Verification items for the finished model (mm, model axes). Give positions to 0.01 mm unless a question says otherwise; leave off trailing zeros. Write each loop counter-clockwise with the first axis right and the second up, starting at its lowest first coordinate (ties: lowest second). Pieces come first, ordered by that corner, then holes. Notation, with made-up numbers: (43.25, -20) - (58.25, -20) arc R20 ccw to (58.25, 12) - close; hole circle Ø7 at (-22.5, -25.5). An arc over 180 degrees is marked (long way). Answer as a JSON object with one key per item and string values. Group by question number.
Item 1: Go/stop test with flat-tipped pins: pin 1 (1.2 mm diameter, centred on x = 2.5, z = -26.5, fed in from -Y); pin 2 (2 mm diameter, centred on x = 1.5, z = -142, fed in from +Y); pin 3 (5 mm diameter, centred on y = 14, z = -33, fed in from -X); pin 4 (2 mm diameter, centred on x = 0.5, z = -36.5, fed in from +Y). Record where each tip stops, or that it passes through.
Item 2: Sectioned sample at B-B, the plane x = 2.8. Record the boundary of the cut face in (y, z), and give its area (3 significant figures).
Item 3: Sectioned sample at D-D, the plane z = 15.5. Record the boundary of the cut face in (x, y).
Item 4: Sectioned sample at A-A, the plane y = 88.9. Record the boundary of the cut face in (x, z), and give its area (3 significant figures).
Item 5: Scan lines: line 1 along Z through (x, y) = (2.35, 88.9); line 2 along Z through (x, y) = (0.6, 25.5); line 3 along Z through (x, y) = (2.65, 115). Record each from-to range of solid material in increasing order. Write a range as [from, to].
Item 6: Draft check along Z on faces 1 (the face through (4.089, 20, -26)), 2 (the face through (2.016, 149.972, 45.235)), 3 (the face through (2.02, 158.74, 43.47)). Enter one of: +Z half, -Z half, draft (parallel to the pull), parting line (faces both ways), or undercut.
Item 7: Sectioned sample at C-C, the plane z = 44.45. Record the boundary of the cut face in (x, y).
```python
from build123d import *

# Parameters (mm, degrees)
F0_R     = 15.621
F0_W     = 5.08
F0_H     = 4.0894
F0_W_2   = 4.826
F1_DEPTH = 4.0894
F2_W     = 5.08
F2_H     = 4.0894
F3_DEPTH = 25.4


with BuildPart() as f1:
    # F0 (on Right) → F1 (new body)
    with BuildSketch(Plane.YZ):
        with BuildLine():
            Line((53.34, -139.7), (114.3, -139.7))
            Line((114.3, -139.7), (114.3, 0))
            Line((114.3, 0), (114.3, 8.769464))
            Line((114.3, 8.769464), (114.3, 80.130536))
            Line((114.3, 80.130536), (114.3, 88.9))
            Line((114.3, 88.9), (-42.671357, 88.9))
            ThreePointArc((-42.671357, 88.9), (-96.063758, -19.892153), (-114.3, -139.7))
            Line((-114.3, -139.7), (-53.34, -139.7))
            Line((-53.34, -139.7), (-48.26, -139.7))
            Line((-48.26, -139.7), (-2.413, -139.7))
            Line((-2.413, -139.7), (2.413, -139.7))
            Line((2.413, -139.7), (48.26, -139.7))
            Line((48.26, -139.7), (53.34, -139.7))
        make_face()
        with Locations((88.9, 44.45)):
            Circle(F0_R, mode=Mode.SUBTRACT)
        with Locations((50.8, -141.7447)):
            Rectangle(F0_W, F0_H)
        with BuildLine():
            Line((114.3, 8.769464), (114.3, 0))
            ThreePointArc((114.3, 0), (158.75, 44.45), (114.3, 88.9))
            Line((114.3, 88.9), (114.3, 80.130536))
            ThreePointArc((114.3, 80.130536), (149.980536, 44.45), (114.3, 8.769464))
        make_face()
        with Locations((0, -141.7447)):
            Rectangle(F0_W_2, F0_H)
        with Locations((-50.8, -141.7447)):
            Rectangle(F0_W, F0_H)
    extrude(amount=F1_DEPTH)

    # F2 (on face) → F3 (cut)
    with BuildSketch(Plane.YZ.offset(4.0894)):
        with Locations((0, -27.4447)):
            Rectangle(F2_W, F2_H)
        with Locations((-25.4, -27.4447)):
            Rectangle(F2_W, F2_H)
    extrude(amount=-F3_DEPTH, mode=Mode.SUBTRACT)


solid = f1.part
```
Geometry check:
{
 "1": {"pin 1": "y = -98.25", "pin 2": "y = 53.34", "pin 3": "x = 0", "pin 4": "y = 114.3"},
 "2": {"outline": "(-114.3, -139.7) - (-53.34, -139.7) - (-53.34, -143.79) - (-48.26, -143.79) - (-48.26, -139.7) - (-2.41, -139.7) - (-2.41, -143.79) - (2.41, -143.79) - (2.41, -139.7) - (48.26, -139.7) - (48.26, -143.79) - (53.34, -143.79) - (53.34, -139.7) - (114.3, -139.7) - (114.3, 0) arc R44.45 ccw to (114.3, 88.9) - (-42.67, 88.9) arc R398.64 ccw to start; hole (-27.94, -29.49) - (-22.86, -29.49) - (-22.86, -25.4) - (-27.94, -25.4) - close; hole (-2.54, -29.49) - (2.54, -29.49) - (2.54, -25.4) - (-2.54, -25.4) - close; hole circle Ø31.24 at (88.9, 44.45); hole (114.3, 8.77) arc R35.68 ccw to (114.3, 80.13) - close", "area": "47,400 mm^2"},
 "3": {"outline": "(0, -83.11) - (4.09, -83.11) - (4.09, 114.3) - (0, 114.3) - close; (0, 135.16) - (4.09, 135.16) - (4.09, 148.03) - (0, 148.03) - close"},
 "4": {"outline": "(0, -139.7) - (4.09, -139.7) - (4.09, 28.83) - (0, 28.83) - close; (0, 60.07) - (4.09, 60.07) - (4.09, 88.9) - (0, 88.9) - close", "area": "807 mm^2"},
 "5": {"line 1": "[-139.7, 28.83], [60.07, 88.9]", "line 2": "[-139.7, 88.9]", "line 3": "[0.01, 8.78], [80.12, 88.89]"},
 "6": {"face 1": "draft", "face 2": "undercut", "face 3": "parting line"},
 "7": {"outline": "(0, -69.54) - (4.09, -69.54) - (4.09, 73.28) - (0, 73.28) - close; (0, 104.52) - (4.09, 104.52) - (4.09, 114.3) - (0, 114.3) - close; (0, 149.98) - (4.09, 149.98) - (4.09, 158.75) - (0, 158.75) - close"}
}
